from build123d import *

# Parameters (mm, degrees)
F1_DEPTH = 1


# Not quite as in the source:
# - ends of sketch curves that miss each other by under 0.0002 mm in the source are joined


with BuildPart() as f1:
    # F0 (on Top) → F1 (new body)
    with BuildSketch(Plane.XY):
        Polygon((-2.198051, 23.051648), (-15.497051, 20.076648), (-15.856751674, 16.3066919689), (-14.8610655684, 16.2861461385), (-14.8610655684, 13.2855074428), (-16.1424234512, 13.311948043), (-18.862051, -15.198352), (0.006949, -31.811352), (20.3729486667, -21.4913521689), (0.507429, 17.711787), (-1.0988393333, 17.0108418244), (-1.0988393333, 20.2840446021), (-0.851051, 20.392648), align=None)
        Polygon((-11.9467116892, 16.2260088921), (-10.468051674, 16.1954969689), (-7.8843876222, 17.3229593784), (-7.8180441633, 17.3229593784), (-7.8180441633, 14.0787076895), (-9.871652, 13.182552), (-11.9467116892, 13.2253702503), align=None, mode=Mode.SUBTRACT)
    extrude(amount=F1_DEPTH)


solid = f1.part
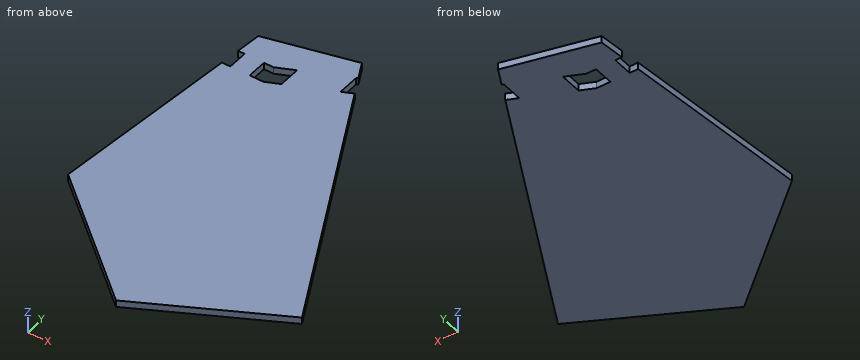
Geometry: final body of the model. Coordinates: model frame, mm. Round coordinates to 2 decimals unless told otherwise and drop trailing zeros. Order: outer loops, then holes, each group sorted by start corner. A loop starts at its lowest first (then second) coordinate and runs counter-clockwise, first axis right, second up. Notation, with made-up numbers: (-5.75, 35) -> (9.25, 35) arc R16 cw to (9.25, 42) -> close; hole circle Ø4 at (27.25, -22.5). An arc over 180 degrees is marked (long way). Put each result on its own line as item: value. Start each with the question number.
Q1. First-contact query: pin 1 (0.5 mm diameter, centred on y = 18, z = 0.5, fed in from +X); pin 2 (4 mm diameter, centred on x = -7, y = -18.5, fed in from -Z). Flat tips, straight axial feed; report the tip coordinate or a pass-through.
Q2. Section A-A on z = 0.2. Return the cut outline in (x, y), and give its area (3 significant figures).
Q3. Section B-B on x = 13. Return the cut outline in (y, z), and give its area (3 significant figures).
Q4. Section C-C on y = -4.5. Return the cut outline in (x, z), and give its area (3 significant figures).
Q5. Line query: probe 1 along Y at (x, z) = (10, 0.55); probe 2 along Y at (x, z) = (3, 0.1); probe 3 along X at (y, z) = (-4, 0.15). Output: solid intervals per line, ascending.
Ans:
1. pin 1: stops at x = -1.1
1. pin 2: stops at z = 0
2. outline: (-18.86, -15.2) -> (0.01, -31.81) -> (20.37, -21.49) -> (0.51, 17.71) -> (-1.1, 17.01) -> (-1.1, 20.28) -> (-0.85, 20.39) -> (-2.2, 23.05) -> (-15.5, 20.08) -> (-15.86, 16.31) -> (-14.86, 16.29) -> (-14.86, 13.29) -> (-16.14, 13.31) -> close; hole (-11.95, 13.23) -> (-9.87, 13.18) -> (-7.82, 14.08) -> (-7.82, 17.32) -> (-7.88, 17.32) -> (-10.47, 16.2) -> (-11.95, 16.23) -> close
2. area: 1,280 mm2
3. outline: (-25.23, 0) -> (-6.94, 0) -> (-6.94, 1) -> (-25.23, 1) -> close
3. area: 18.3 mm2
4. outline: (-17.84, 0) -> (11.76, 0) -> (11.76, 1) -> (-17.84, 1) -> close
4. area: 29.6 mm2
5. probe 1: y = -26.75 to -1.02
5. probe 2: y = -30.29 to 12.79
5. probe 3: x = -17.79 to 11.51
